Autodesk Inventor part; units mm, degrees
ref_plane "YZ Plane" through (0, 0, 0) normal (1, 0, 0) x (0, 1, 0)
ref_plane "XZ Plane" through (0, 0, 0) normal (0, 1, 0) x (-1, 0, 0)
ref_plane "XY Plane" through (0, 0, 0) normal (0, 0, 1) x (1, 0, 0)
sketch "Sketch1" plane through (0, 0, 0) normal (0, 0, 1) x (1, 0, 0)
  line L0 (-50.8, -38.1) -> (50.8, -38.1)
  line L1 (50.8, -38.1) -> (50.8, 38.1)
  line L2 (50.8, 38.1) -> (-50.8, 38.1)
  line L3 (-50.8, 38.1) -> (-50.8, -38.1)
  line L4 (-50.8, -38.1) -> (50.8, 38.1) construction
  line L5 (50.8, -38.1) -> (-50.8, 38.1) construction
  line L6 (-38.1, -25.4) -> (38.1, -25.4)
  line L7 (38.1, -25.4) -> (38.1, 25.4)
  line L8 (38.1, 25.4) -> (-38.1, 25.4)
  line L9 (-38.1, 25.4) -> (-38.1, -25.4)
  line L10 (-38.1, -25.4) -> (38.1, 25.4) construction
  line L11 (38.1, -25.4) -> (-38.1, 25.4) construction
  circle A0 centre (-38.1, 25.4) radius 6.35
  circle A1 centre (38.1, 25.4) radius 6.35
  circle A2 centre (-38.1, -25.4) radius 6.35
  circle A3 centre (38.1, -25.4) radius 6.35
  circle A4 centre (0, -12.7) radius 6.0944
  point P0 (0, 0)
  dimension "d0" = 101.6
  dimension "d1" = 76.2
  dimension "d2" = 76.2
  dimension "d3" = 50.8
  dimension "d4" = 12.7
  dimension "d7" = 50.8
extrude "Extrusion1" add sketch "Sketch1" along normal blind 25.4 contours L3 L2 L1 L0 | A2 L9 A0 L8 A1 L7 A3 L6
sketch "Sketch2" plane through (50.8, -38.1, 0) normal (1, 0, 0) x (0, 0, -1)
  line L0 (0, 76.2) -> (0, 0)
  line L1 (0, 0) -> (-25.4, 0)
  line L2 (-25.4, 0) -> (-25.4, 25.4)
  line L3 (-25.4, 25.4) -> (0, 25.4)
  line L4 (0, 25.4) -> (0, 0)
  line L5 (0, 76.2) -> (-25.4, 76.2)
  point P0 (0, 38.1)
  point P1 (0, 25.4)
  dimension "d8" = 25.4
extrude "Extrusion2" add sketch "Sketch2" along normal blind 101.6
mirror "Mirror1" about plane through (0, 0, 0) normal (1, 0, 0) of "Extrusion2"
sketch "Sketch3" plane through (50.8, -12.7, 25.4) normal (0, 1, 0) x (1, 0, 0)
  line L0 (0, 0) -> (-101.6, 0)
  line L1 (-50.8, 0) -> (-50.8, 25.4) construction
  line L2 (-203.2, 25.4) -> (-203.2, 0)
  line L3 (-203.2, 12.7) -> (101.6, 12.7) construction
  line L4 (101.6, 0) -> (101.6, 25.4)
  circle A0 centre (76.2, 12.7) radius 6.35
  circle A1 centre (-177.8, 12.7) radius 6.35
  dimension "d11" = 12.7
  dimension "d12" = 127
extrude "Extrusion3" cut sketch "Sketch3" against normal through all
properties part number "center block"
Geometry check sheet. Reference: the model listing, model coordinates, mm. A direction names the side the tool comes from. Coordinates: 2 decimals unless noted, no trailing zeros. Write each loop counter-clockwise with the first axis right and the second up, starting at its lowest first coordinate (ties: lowest second). Pieces come first, ordered by that corner, then holes. Notation, with made-up numbers: M -21.5,42 L -9.5,42 A7 ccw -9.5,54 Z; hole C -37.5,39 d6. An arc over 180 degrees is marked long. One line per item, written item: value. Start each with the question number.
(1) Sectioned sample at C-C, the plane z = 12.7. Enter the section's corners in (x, y), and give its area (3 significant figures).
(2) Scan lines: line 1 along X through (y, z) = (25.4, 12.5); line 2 along Y through (x, z) = (38.1, 18.25); line 3 along X through (y, z) = (-22, 23.75). Record each from-to range of solid material in increasing order. Write a range as [from, to].
(3) Depth check by flat-ended pin: pin 1 (7.5 mm diameter, centred on x = 38.1, y = 25.4, fed in from -Z); pin 2 (5 mm diameter, centred on y = 21, z = 14, fed in from -X); pin 3 (12.5 mm diameter, centred on x = 77, z = 14.5, fed in from +Y); pin 4 (1.5 mm diameter, centred on y = -2, z = 15, fed in from +X). Enter the tip coordinate at first touch or a pass-through.
(4) Sectioned sample at A-A, the plane y = -25.4. Enter the section's corners in (x, z).
(5) Tool access check on faces 5 (the face through (-32.234, -22.968, 12.522)), 6 (the face through (50.8, 12, 13)), 7 (the face through (-50.8, 13, 13)). Record the directions out of +Z, -Z, +X, -X, +Y, -Y that give a thin tool (end or side, any length) a straight path to the whole face; none if there is none.
(6) Sectioned sample at B-B, the plane x = 38.1. Enter the section's corners in (y, z).
(7) Sectioned sample at D-D, the plane x = -127. Enter the section's corners in (y, z), and give its area (3 significant figures).
(8) Release check for a two-part mould opening along Z. For faces 1 (the face through (-152.4, -25, 13)), 2 (the face through (133.057, -25.222, 10.793)), 3 (the face through (-121.134, -25.222, 15.132)), 4 (the face through (2, -1, 0)) record: released by +Z, released by -Z, zero draft, split by the parting line, or undercut.
Filled sheet:
1. outline: M -152.4,-38.1 L -133.35,-38.1 L -133.35,-12.7 L -152.4,-12.7 Z; M -120.65,-38.1 L 120.65,-38.1 L 120.65,-12.7 L 50.8,-12.7 L 50.8,38.1 L -50.8,38.1 L -50.8,-12.7 L -120.65,-12.7 Z; M 133.35,-38.1 L 152.4,-38.1 L 152.4,-12.7 L 133.35,-12.7 Z; hole C -38.1,-25.4 d12.7; hole C -38.1,25.4 d12.7; hole C 0,-12.7 d12.19; hole C 38.1,-25.4 d12.7; hole C 38.1,25.4 d12.7
1. area: 11,600 mm²
2. line 1: [-50.8, -44.45], [-31.75, 31.75], [44.45, 50.8]
2. line 2: [-38.1, -31.75], [-19.05, 19.05], [31.75, 38.1]
2. line 3: [-152.4, -43.46], [-32.74, 32.74], [43.46, 152.4]
3. pin 1: through
3. pin 2: x = -50.8
3. pin 3: y = -12.7
3. pin 4: x = 50.8
4. outline: M -152.4,0 L -44.45,0 L -44.45,25.4 L -152.4,25.4 Z; M -31.75,0 L 31.75,0 L 31.75,25.4 L -31.75,25.4 Z; M 44.45,0 L 152.4,0 L 152.4,25.4 L 44.45,25.4 Z; hole C -127,12.7 d12.7; hole C 127,12.7 d12.7
5. face 5: +Z, -Z
5. face 6: +Z, -Z, +X, +Y
5. face 7: +Z, -Z, -X, +Y
6. outline: M -38.1,0 L -31.75,0 L -31.75,25.4 L -38.1,25.4 Z; M -19.05,0 L 19.05,0 L 19.05,25.4 L -19.05,25.4 Z; M 31.75,0 L 38.1,0 L 38.1,25.4 L 31.75,25.4 Z
7. outline: M -38.1,0 L -12.7,0 L -12.7,6.35 L -38.1,6.35 Z; M -38.1,19.05 L -12.7,19.05 L -12.7,25.4 L -38.1,25.4 Z
7. area: 323 mm²
8. face 1: zero draft
8. face 2: undercut
8. face 3: undercut
8. face 4: released by -Z
